For this review, take the finished solid that the model builds, in its own axes (mm). A direction names the side the tool comes from. Give positions to 0.01 mm unless a question says otherwise; leave off trailing zeros. Loops run counter-clockwise (first coordinate to the right, second up) from the corner with the lowest first, then second, coordinate; pieces in that order, holes last.
Autodesk Inventor part; units mm, degrees
ref_plane "YZ Plane" through (0, 0, 0) normal (1, 0, 0) x (0, 1, 0)
ref_plane "XZ Plane" through (0, 0, 0) normal (0, 1, 0) x (-1, 0, 0)
ref_plane "XY Plane" through (0, 0, 0) normal (0, 0, 1) x (1, 0, 0)
sketch "Sketch1" plane through (0, 0, 0) normal (0, 0, 1) x (1, 0, 0)
  line L0 (-27, 20) -> (27, 20)
  line L1 (27, 20) -> (27, -20)
  line L2 (27, -20) -> (-27, -20)
  line L3 (-27, -20) -> (-27, 20)
  line L4 (-27, 20) -> (27, -20) construction
  line L5 (27, 20) -> (-27, -20) construction
  point P0 (0, 0)
  dimension "d0" = 54
  dimension "d1" = 40
extrude "Extrusion1" add sketch "Sketch1" along normal blind 12
sketch "Sketch2" plane through (0, 0, 12) normal (0, 0, 1) x (1, 0, 0)
  line L0 (-24, -20) -> (24, -20)
  line L1 (24, -20) -> (24, 20)
  line L2 (24, 20) -> (-24, 20)
  line L3 (-24, 20) -> (-24, -20)
  line L4 (-24, -20) -> (24, 20) construction
  line L5 (24, -20) -> (-24, 20) construction
  point P0 (0, 0)
  dimension "d4" = 48
  dimension "d5" = 40
extrude "Extrusion2" cut sketch "Sketch2" against normal blind 9
sketch "Sketch3" plane through (-24, -20, 12) normal (1, 0, 0) x (0, 0, -1)
  line L0 (9, 0) -> (0, 0)
  line L1 (0, 0) -> (0, 5)
  line L2 (0, 40) -> (0, 0)
  line L3 (0, 5) -> (0, 35)
  line L4 (0, 5) -> (4, 5)
  line L5 (0, 0) -> (0, 40)
  line L6 (0, 5) -> (4, 5) construction
  line L7 (0, 35) -> (4, 35)
  line L8 (0, 35) -> (4, 35) construction
  line L9 (1.2287, 35) -> (2.6144, 37.4)
  line L10 (2.6144, 37.4) -> (5.3856, 37.4)
  line L11 (5.3856, 37.4) -> (6.7713, 35)
  line L12 (6.7713, 35) -> (5.3856, 32.6)
  line L13 (5.3856, 32.6) -> (2.6144, 32.6)
  line L14 (2.6144, 32.6) -> (1.2287, 35)
  line L15 (1.2287, 5) -> (2.6144, 7.4)
  line L16 (2.6144, 7.4) -> (5.3856, 7.4)
  line L17 (5.3856, 7.4) -> (6.7713, 5)
  line L18 (6.7713, 5) -> (5.3856, 2.6)
  line L19 (5.3856, 2.6) -> (2.6144, 2.6)
  line L20 (2.6144, 2.6) -> (1.2287, 5)
  line L21 (9, 40) -> (9, 0) construction
  line L22 (9, 0) -> (9, 40) construction
  point P0 (12, 20)
  dimension "d8" = 5
  dimension "d9" = 30
  dimension "d10" = 180
  dimension "d11" = 4
  dimension "d12" = 0
  dimension "d13" = 4
  dimension "d14" = 0
  dimension "d15" = 4.8
  dimension "d16" = 4.8
extrude "Extrusion3" cut sketch "Sketch3" against normal blind 2
sketch "Sketch4" plane through (24, -20, 12) normal (-1, 0, 0) x (0, 0, 1)
  line L0 (-9, 0) -> (-9, 5)
  line L1 (-9, 40) -> (-9, 0)
  line L2 (-9, 5) -> (-9, 20)
  line L3 (-9, 20) -> (-1, 20)
  line L4 (-9, 5) -> (-5, 5)
  line L5 (-9, 5) -> (-5, 5) construction
  line L6 (-7.7713, 5) -> (-6.3856, 7.4)
  line L7 (-6.3856, 7.4) -> (-3.6144, 7.4)
  line L8 (-3.6144, 7.4) -> (-2.2287, 5)
  line L9 (-2.2287, 5) -> (-3.6144, 2.6)
  line L10 (-3.6144, 2.6) -> (-6.3856, 2.6)
  line L11 (-6.3856, 2.6) -> (-7.7713, 5)
  line L12 (-7.7713, 35) -> (-6.3856, 32.6)
  line L13 (-6.3856, 32.6) -> (-3.6144, 32.6)
  line L14 (-3.6144, 32.6) -> (-2.2287, 35)
  line L15 (-2.2287, 35) -> (-3.6144, 37.4)
  line L16 (-3.6144, 37.4) -> (-6.3856, 37.4)
  line L17 (-6.3856, 37.4) -> (-7.7713, 35)
  point P0 (-12, 20)
  dimension "d19" = 5
  dimension "d20" = 15
  dimension "d21" = 180
  dimension "d22" = 8
  dimension "d23" = 90
  dimension "d24" = 4
  dimension "d25" = 0
  dimension "d26" = 4.8
extrude "Extrusion4" cut sketch "Sketch4" against normal blind 2
sketch "Sketch6" plane through (24, -20, 12) normal (-1, 0, 0) x (0, 0, 1)
  line L0 (-9, 0) -> (-9, 5)
  line L1 (-9, 0) -> (-4, 0) construction
  line L2 (-9, 5) -> (-5, 5)
  line L3 (-9, 5) -> (-9, 20)
  line L4 (-9, 5) -> (6, 5) construction
  line L5 (-9, 20) -> (-1, 20)
  circle A0 centre (-5, 5) radius 1.35
  circle A1 centre (-5, 35) radius 1.35
  point P0 (-12, 20)
  dimension "d29" = 5
  dimension "d30" = 90
  dimension "d31" = 4
  dimension "d32" = 90
  dimension "d33" = 15
  dimension "d34" = 90
  dimension "d35" = 8
  dimension "d36" = 90
  dimension "d37" = 2.7
extrude "Extrusion5" cut sketch "Sketch6" against normal up to surface (3 mm away)
sketch "Sketch7" plane through (-27, -20, 0) normal (-1, 0, 0) x (0, 0, 1)
  line L0 (12, 0) -> (12, 40)
  line L1 (12, 0) -> (12, 5)
  line L2 (12, 0) -> (17, 0) construction
  line L3 (12, 5) -> (8, 5)
  line L4 (12, 5) -> (12, 20)
  line L5 (12, 5) -> (27, 5) construction
  line L6 (12, 20) -> (0, 20)
  circle A0 centre (8, 5) radius 1.35
  circle A1 centre (8, 35) radius 1.35
  dimension "d40" = 5
  dimension "d41" = 90
  dimension "d42" = 4
  dimension "d43" = 90
  dimension "d44" = 15
  dimension "d45" = 90
  dimension "d46" = 2.7
extrude "Extrusion6" cut sketch "Sketch7" against normal up to surface (3 mm away)
sketch "Sketch8" plane through (0, 0, 3) normal (0, 0, 1) x (1, 0, 0)
  line L0 (24, -20) -> (-24, -20)
  line L1 (-24, -20) -> (-21, -20)
  line L2 (-24, -20) -> (-21, -20) construction
  line L3 (-24, 20) -> (24, 20)
  line L4 (-21, -20) -> (-21, -17)
  line L5 (-21, -20) -> (-18, -20) construction
  line L6 (-21, -17) -> (21, -17) construction
  line L7 (21, -17) -> (21, 17) construction
  line L8 (21, 17) -> (-21, 17)
  line L9 (-21, 17) -> (-21, -17)
  line L10 (21, -17) -> (21, -15)
  line L11 (21, -17) -> (23, -17) construction
  line L12 (21, -17) -> (19, -17)
  line L13 (21, -17) -> (23, -17) construction
  line L14 (21, -15) -> (41, -15) construction
  line L15 (-21, 17) -> (-21, 15)
  line L16 (21, 17) -> (-21, -17)
  line L17 (-21, 17) -> (21, -17)
  line L18 (-19.7416, -18.5545) -> (22.2584, 15.4455) construction
  line L19 (22.2584, 15.4455) -> (19.7416, 18.5545)
  line L20 (19.7416, 18.5545) -> (-22.2584, -15.4455) construction
  line L21 (-22.2584, -15.4455) -> (-19.7416, -18.5545)
  line L22 (-19.7416, -18.5545) -> (19.7416, 18.5545) construction
  line L23 (22.2584, 15.4455) -> (-22.2584, -15.4455) construction
  line L24 (-22.2584, 15.4455) -> (19.7416, -18.5545) construction
  line L25 (19.7416, -18.5545) -> (22.2584, -15.4455)
  line L26 (22.2584, -15.4455) -> (-19.7416, 18.5545) construction
  line L27 (-19.7416, 18.5545) -> (-22.2584, 15.4455)
  line L28 (-22.2584, 15.4455) -> (22.2584, -15.4455) construction
  line L29 (19.7416, -18.5545) -> (-19.7416, 18.5545) construction
  line L30 (0, -2.5732) -> (-17.8214, -17)
  line L31 (0, -2.5732) -> (17.8214, -17)
  line L32 (17.8214, -17) -> (-17.8214, -17)
  line L33 (24, -20) -> (-24, -20) construction
  line L34 (24, 20) -> (24, -20) construction
  line L35 (-24, 20) -> (24, 20) construction
  line L36 (-24, -20) -> (-24, 20) construction
  line L37 (-21, 0) -> (21, 0) construction
  line L38 (0, 17) -> (0, -17) construction
  line L39 (0, 2.5732) -> (-17.8214, 17)
  line L40 (0, 2.5732) -> (17.8214, 17)
  line L41 (17.8214, 17) -> (-17.8214, 17)
  line L42 (3.1786, 0) -> (21, -14.4268)
  line L43 (3.1786, 0) -> (21, 14.4268)
  line L44 (21, 14.4268) -> (21, -14.4268)
  line L45 (-3.1786, 0) -> (-21, -14.4268)
  line L46 (-3.1786, 0) -> (-21, 14.4268)
  line L47 (-21, 14.4268) -> (-21, -14.4268)
  point P0 (0, 0)
  dimension "d49" = 3
  dimension "d50" = 0
  dimension "d52" = 3
  dimension "d53" = 90
  dimension "d54" = 42
  dimension "d55" = 34
  dimension "d56" = 2
  dimension "d57" = 90
  dimension "d58" = 2
  dimension "d59" = 180
  dimension "d64" = 2
  dimension "d65" = 4
  dimension "d66" = 54.037
  dimension "d67" = 4
  dimension "d68" = 54.037
extrude "Extrusion7" cut sketch "Sketch8" against normal up to surface (3 mm away) contours L40 L39 L8 | L9 L46 L45 | L31 L32 L30 | L43 L44 L42
fillet "Fillet1" radius 2 12 edges at (-17.8214, -17, 1.5) (-21, -14.4268, 1.5) (-21, 14.4268, 1.5) (-17.8214, 17, 1.5) (21, 14.4268, 1.5) (17.8214, 17, 1.5) (0, 2.5732, 1.5) (-3.1786, 0, 1.5) (3.1786, 0, 1.5) (0, -2.5732, 1.5) (21, -14.4268, 1.5) (17.8214, -17, 1.5)
properties part number "upper_leg_spacer"
Q1. Machinability: for faces 1 (the flat face through (-24.99, -13.82, 10.09)), 2 (the flat face through (-24, 0, 8)), 3 (the cylindrical face through (-26.507, 16.138, 8.726)), 4 (the cylindrical face through (-4.357, 0.025, 1.479)), which of the approach directions +Z, -Z, +X, -X, +Y, -Y give a long, thin tool a straight path to every point of the face, cutting with its end or side? Answer none if there is none.
Answers:
face 1: none
face 2: +Z, +Y, -Y
face 3: -X
face 4: +Z, -Z
Q2. For probe 1 along Y at (x, z) = (26.5, 7); probe 2 along X at (y, z) = (3.5, 9.25); probe 3 along Y at (x, z) = (11.5, 2.5), list the stretches that pass through material, from the lowest coordinate up.
Answers:
probe 1: y = -20 to -16.35, -13.65 to 13.65, 16.35 to 20
probe 2: x = -27 to -24, 24 to 27
probe 3: y = -20 to -17, -11.88 to -6.74, 6.74 to 11.88, 17 to 20
Q3. For pin 1 Ø2 at (y, z) = (-15, 8) entering from -X; pin 2 Ø10 at (x, y) = (-2, 6.5) entering from +Z, all flat-tipped, find the tip position at first contact; note any pin that passes through.
Answers:
pin 1: stops at x = 26
pin 2: stops at z = 3
Q4. Consider section A-A on y = 5.5. Give the boundary of the cut face in (x, z).
Answers:
outline: (-27, 0) - (-21, 0) - (-21, 3) - (-24, 3) - (-24, 12) - (-27, 12) - close; (-9.97, 0) - (-3.62, 0) - (-3.62, 3) - (-9.97, 3) - close; (3.62, 0) - (9.97, 0) - (9.97, 3) - (3.62, 3) - close; (21, 0) - (27, 0) - (27, 12) - (24, 12) - (24, 3) - (21, 3) - close
Q5. Consider section C-C on x = 10. Give the boundary of the cut face in (y, z).
Answers:
outline: (-20, 0) - (-17, 0) - (-17, 3) - (-20, 3) - close; (-10.67, 0) - (-5.52, 0) - (-5.52, 3) - (-10.67, 3) - close; (5.52, 0) - (10.67, 0) - (10.67, 3) - (5.52, 3) - close; (17, 0) - (20, 0) - (20, 3) - (17, 3) - close
Q6. Consider section B-B on x = -20. Give the boundary of the cut face in (y, z), plus the area to 3 significant figures.
Answers:
outline: (-20, 0) - (-11.97, 0) - (-11.97, 3) - (-20, 3) - close; (11.97, 0) - (20, 0) - (20, 3) - (11.97, 3) - close
area: 48.2 mm2
Q7. Consider section D-D on y = 18. Give the boundary of the cut face in (x, z), plus the area to 3 significant figures.
Answers:
outline: (-27, 0) - (27, 0) - (27, 12) - (24, 12) - (24, 3) - (-24, 3) - (-24, 12) - (-27, 12) - close
area: 216 mm2
Q8. Mouldability with a two-part tool opening along X and no side actions: class faces 5 (the flat face through (0, 0, 0)), 6 (the flat face through (27, 0, 6)), 7 (the flat face through (-21, 0, 2)) as +X half, -X half, draft (parallel to the pull), parting line (faces both ways), or undercut.
Answers:
face 5: draft
face 6: +X half
face 7: undercut
